from build123d import *

# Parameters (mm, degrees)
SKETCH_1_R      = 6
EXTRUDE_1_DEPTH = 38
SKETCH_2_R      = 3.5
EXTRUDE_2_DEPTH = 3
SKETCH_4_R      = 3.5
EXTRUDE_3_DEPTH = 10
SKETCH_6_R      = 7.5
EXTRUDE_5_DEPTH = 4.5
CHAMFER_1_SIZE  = 1.8


with BuildPart() as part:
    # Эскиз1 → Бобышка-Вытянуть1 (new body)
    with BuildSketch(Plane.XY):
        Circle(SKETCH_1_R)
    extrude(amount=EXTRUDE_1_DEPTH)

    # Эскиз2 → Бобышка-Вытянуть2 (add)
    with BuildSketch(Plane.XY.offset(38)):
        Circle(SKETCH_2_R)
    extrude(amount=EXTRUDE_2_DEPTH)

    # Эскиз4 → Бобышка-Вытянуть3 (add)
    with BuildSketch(Plane(origin=(0, 0, 0), x_dir=(-1, 0, 0), z_dir=(0, 0, -1))):
        Circle(SKETCH_4_R)
    extrude(amount=EXTRUDE_3_DEPTH)

    # Эскиз6 → Бобышка-Вытянуть5 (add)
    with BuildSketch(Plane(origin=(0, 0, 0), x_dir=(-1, 0, 0), z_dir=(0, 0, -1))):
        Circle(SKETCH_6_R)
    extrude(amount=-EXTRUDE_5_DEPTH)

    # Фаска1
    chamfer_1_edges = [part.edges().sort_by_distance(p)[0] for p in [
        (-6, 0, 38),
    ]]
    chamfer(chamfer_1_edges, length=CHAMFER_1_SIZE)


solid = part.part
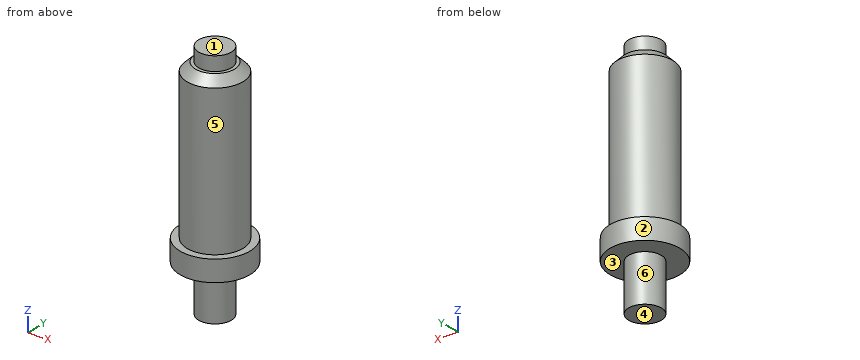
Verification items for the finished model (mm, model axes). Face numbers are marked on the shaded views. A direction names the side the tool comes from. Coordinates: 2 decimals unless noted, no trailing zeros. Order: outer loops, then holes, each group sorted by start corner. A loop starts at its lowest first (then second) coordinate and runs counter-clockwise, first axis right, second up. Notation, with made-up numbers: M -37.5,63.5 L -30.5,63.5 A17 ccw -30.5,70.5 Z; hole C -28.75,-18 d5. An arc over 180 degrees is marked long. Return JSON: item names as keys, results as strings.
1) Gauge pin test, flat ends, axial feed: pin 1 (2 mm diameter, centred on x = -5.5, z = 4.5, fed in from -Y); pin 2 (5 mm diameter, centred on x = -6, z = 19.5, fed in from +Y); pin 3 (4 mm diameter, centred on y = -5, z = 18, fed in from +X). Record the tip position at first contact, or that the pin passes through.
Answer list:
{"pin 1": "y = -6", "pin 2": "y = 4.87", "pin 3": "x = 5.2"}
2) Release check for a two-part mould opening along Z. For the marked faces 1, 2 and 3 record: +Z half, -Z half, draft (parallel to the pull), parting line (faces both ways), or undercut.
Answer list:
{"face 1": "+Z half", "face 2": "draft", "face 3": "-Z half"}
3) Thickness scan on L1, parallel to Z at x = -4, y = -1; L2, parallel to Y at x = 0, z = 26; L3, parallel to Z at x = -4.5, y = -5.75. Record the ranges inside material, lowest first. Write a range as [from, to].
Answer list:
{"L1": "[0, 38]", "L2": "[-6, 6]", "L3": "[0, 4.5]"}
4) Cross-section at C-C, the plane z = 3.5. Record the boundary of the cut face in (x, y).
Answer list:
{"outline": "C 0,0 d15"}
5) Cross-section at A-A, the plane x = 0. Record the boundary of the cut face in (y, z), and give its area (3 significant figures).
Answer list:
{"outline": "M -7.5,0 L -3.5,0 L -3.5,-10 L 3.5,-10 L 3.5,0 L 7.5,0 L 7.5,4.5 L 6,4.5 L 6,36.2 L 4.2,38 L 3.5,38 L 3.5,41 L -3.5,41 L -3.5,38 L -4.2,38 L -6,36.2 L -6,4.5 L -7.5,4.5 Z", "area": "557 mm2"}
6) Cross-section at D-D, the plane z = 15. Record the boundary of the cut face in (x, y), and give its area (3 significant figures).
Answer list:
{"outline": "C 0,0 d12", "area": "113 mm2"}
7) Access from +Z, -Z, +X, -X, +Y, -Y to the whole of each face (thin tool, end or side, straight path). Record for the marked faces 4, 5 and 6.
Answer list:
{"face 4": "-Z, +X, -X, +Y, -Y", "face 5": "+Z", "face 6": "-Z"}
